Can you work these out from the model? Positions are in its coordinate system, mm. Face numbers are marked on the shaded views. A direction names the side the tool comes from. Give positions to 0.01 mm unless a question says otherwise; leave off trailing zeros. Write each loop counter-clockwise with the first axis right and the second up, starting at its lowest first coordinate (ties: lowest second). Pieces come first, ordered by that corner, then holes.
```python
from build123d import *

# Parameters (mm, degrees)
SKETCH1_W                                       = 25
SKETCH1_H                                       = 25
BOSS_EXTRUDE1_DEPTH                             = 2.5
SKETCH2_W                                       = 25
SKETCH2_H                                       = 3
BOSS_EXTRUDE2_DEPTH                             = 13.5
SKETCH10_R                                      = 2
CUT_EXTRUDE1_DEPTH                              = 26
SKETCH10_3_R                                    = 0.8
CUT_EXTRUDE2_DEPTH                              = 26
FILLET1_R                                       = 0.762
CHAMFER1_SIZE                                   = 5
CSK_FOR_M2_FLAT_HEAD_MACHINE_SCREW1_D           = 2.4
CSK_FOR_M2_FLAT_HEAD_MACHINE_SCREW1_CSINK_D     = 4.4
CSK_FOR_M2_FLAT_HEAD_MACHINE_SCREW1_CSINK_ANGLE = 90


with BuildPart() as part:
    # Sketch1 → Boss-Extrude1 (new body)
    with BuildSketch(Plane.XY):
        Rectangle(SKETCH1_W, SKETCH1_H)
    extrude(amount=BOSS_EXTRUDE1_DEPTH)

    # Sketch2 → Boss-Extrude2 (add)
    with BuildSketch(Plane(origin=(0, 0, 0), x_dir=(-1, 0, 0), z_dir=(0, 0, -1))):
        with Locations((0, 11)):
            Rectangle(SKETCH2_W, SKETCH2_H)
        with Locations((0, -11)):
            Rectangle(SKETCH2_W, SKETCH2_H)
    extrude(amount=BOSS_EXTRUDE2_DEPTH)

    # Sketch10 → Cut-Extrude1 (cut, through all)
    with BuildSketch(Plane.XZ.offset(12.5)):
        with Locations((5.5, -4.5)):
            Circle(SKETCH10_R)
    extrude(amount=-CUT_EXTRUDE1_DEPTH, mode=Mode.SUBTRACT)

    # Sketch10<3> → Cut-Extrude2 (cut, through all)
    with BuildSketch(Plane.XZ.offset(12.5)):
        with Locations((9.5, -8.5)):
            Circle(SKETCH10_3_R)
    extrude(amount=-CUT_EXTRUDE2_DEPTH, mode=Mode.SUBTRACT)

    # Fillet1
    fillet1_edges = [part.edges().sort_by_distance(p)[0] for p in [
        (0, 9.5, 0),
        (0, -9.5, 0),
    ]]
    fillet(fillet1_edges, radius=FILLET1_R)

    # Chamfer1
    chamfer1_edges = [part.edges().sort_by_distance(p)[0] for p in [
        (12.5, 11, -13.5),
        (12.5, -11, -13.5),
    ]]
    chamfer(chamfer1_edges, length=CHAMFER1_SIZE)

    # CSK for M2 Flat Head Machine Screw1 (through all)
    with Locations(Plane(origin=(0, 0, 0), x_dir=(-1, 0, 0), z_dir=(0, 0, -1))):
        with Locations((0, 4), (0, -4), (-4, 0)):
            CounterSinkHole(CSK_FOR_M2_FLAT_HEAD_MACHINE_SCREW1_D / 2, CSK_FOR_M2_FLAT_HEAD_MACHINE_SCREW1_CSINK_D / 2, counter_sink_angle=CSK_FOR_M2_FLAT_HEAD_MACHINE_SCREW1_CSINK_ANGLE)


solid = part.part
```
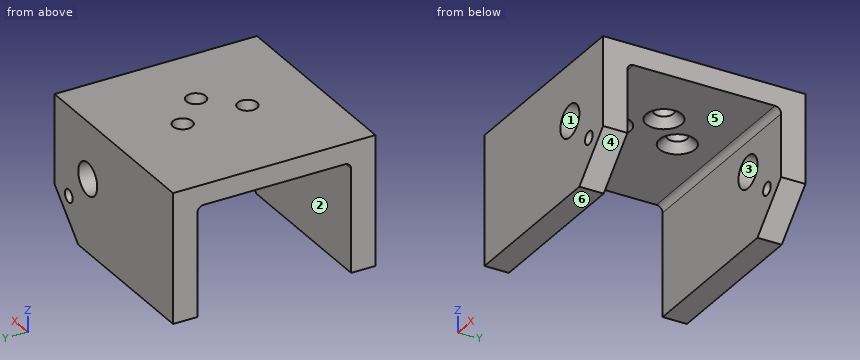
1) For pin 1 Ø6 at (x, y) = (-8, 0) entering from -Z; pin 2 Ø2.5 at (x, z) = (5.5, -4.5) entering from -Y; pin 3 Ø3 at (x, y) = (0, -4) entering from +Z; pin 4 Ø3 at (x, y) = (4, 0) entering from -Z, each with a flat end and sliding along its axis, tell me the tip position at first contact or that it passes through.
Values follow:
pin 1: stops at z = 0
pin 2: passes through
pin 3: stops at z = 2.5
pin 4: stops at z = 0.7
2) Suppose I cut it at D-D on z = -10. Write out the boundary of the cut face in (x, y), plus the area to 3 significant figures.
Values follow:
outline: (-12.5, -12.5) - (11, -12.5) - (11, -9.5) - (-12.5, -9.5) - close; (-12.5, 9.5) - (11, 9.5) - (11, 12.5) - (-12.5, 12.5) - close
area: 141 mm2
3) Please list where these lines run through material, in increasing order: L1, parallel to Y at x = 0, z = 1.3; L2, parallel to X at y = 0, z = 1.5; L3, parallel to Y at x = -6.75, z = -1.5.
Values follow:
L1: y = -12.5 to -5.2, -2.8 to 2.8, 5.2 to 12.5
L2: x = -12.5 to 2.8, 5.2 to 12.5
L3: y = -12.5 to -9.5, 9.5 to 12.5
4) Suppose I cut it at B-B on x = 0. Write out the boundary of the cut face in (y, z).
Values follow:
outline: (-12.5, -13.5) - (-9.5, -13.5) - (-9.5, -0.76) arc R0.76 cw to (-8.74, 0) - (-6.2, 0) - (-5.2, 1) - (-5.2, 2.5) - (-12.5, 2.5) - close; (-2.8, 1) - (-1.8, 0) - (1.8, 0) - (2.8, 1) - (2.8, 2.5) - (-2.8, 2.5) - close; (5.2, 1) - (6.2, 0) - (8.74, 0) arc R0.76 cw to (9.5, -0.76) - (9.5, -13.5) - (12.5, -13.5) - (12.5, 2.5) - (5.2, 2.5) - close
5) Suppose I cut it at A-A on y = 4. Write out the boundary of the cut face in (x, z), plus the area to 3 significant figures.
Values follow:
outline: (-12.5, 0) - (-2.2, 0) - (-1.2, 1) - (-1.2, 2.5) - (-12.5, 2.5) - close; (1.2, 1) - (2.2, 0) - (12.5, 0) - (12.5, 2.5) - (1.2, 2.5) - close
area: 55.5 mm2
6) If we mould it in two halves opening along X, with no side actions, what happens to the marked faces 1, 2, 3 and 4? For each: +X half, -X half, draft (parallel to the pull), parting line (faces both ways), or undercut.
Values follow:
face 1: undercut
face 2: draft
face 3: undercut
face 4: +X half
7) Suppose I cut it at C-C on z = -4.5. Write out the boundary of the cut face in (x, y).
Values follow:
outline: (-12.5, -12.5) - (3.5, -12.5) - (3.5, -9.5) - (-12.5, -9.5) - close; (-12.5, 9.5) - (3.5, 9.5) - (3.5, 12.5) - (-12.5, 12.5) - close; (7.5, -12.5) - (12.5, -12.5) - (12.5, -9.5) - (7.5, -9.5) - close; (7.5, 9.5) - (12.5, 9.5) - (12.5, 12.5) - (7.5, 12.5) - close
8) For the marked faces 5 and 6, which set-ups out of +Z, -Z, +X, -X, +Y, -Y let a thin tool reach every point of the face, with its end or its side?
Values follow:
face 5: -Z, +X, -X
face 6: -Z, +X, -X, +Y, -Y
